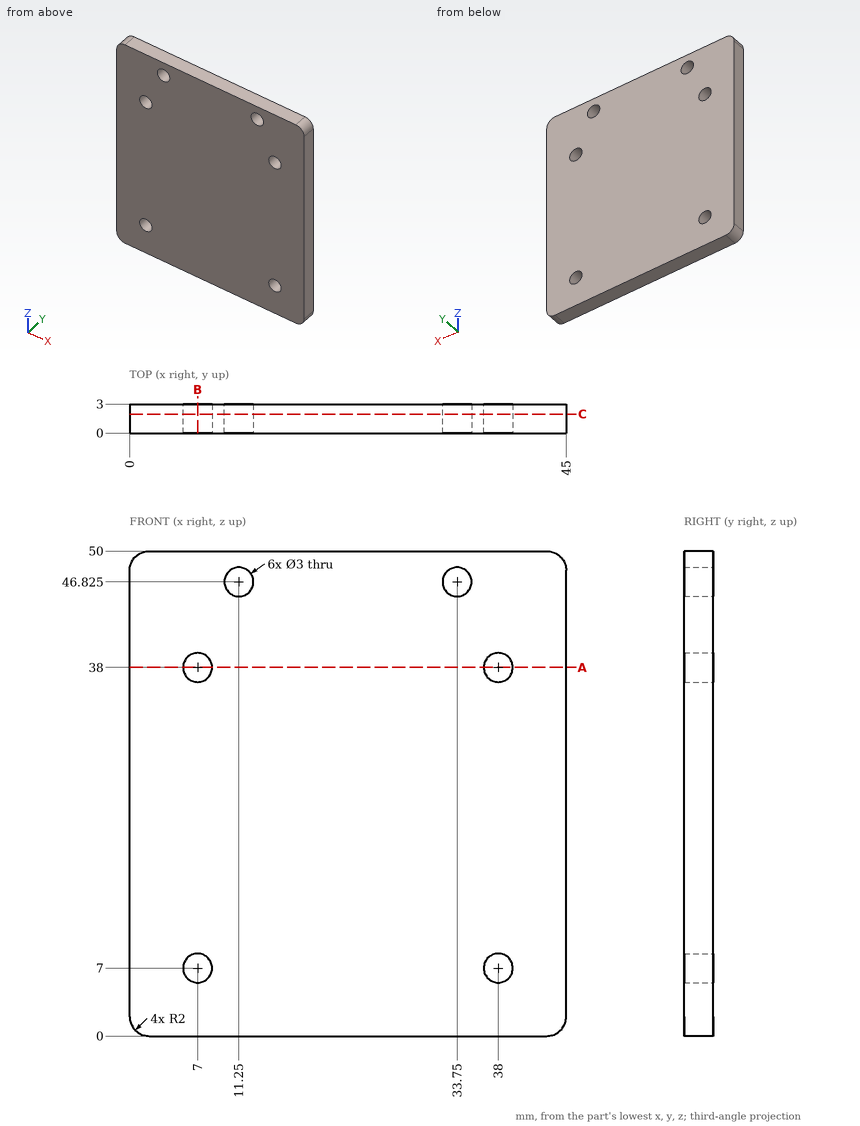
Can you work these out from the drawing? Everything is in mm from the part's minimum corner. Coordinates: 2 decimals unless noted, no trailing zeros. Loops run counter-clockwise (first coordinate to the right, second up) from the corner with the lowest first, then second, coordinate; pieces in that order, holes last. Notation, with made-up numbers: (-20, -33.5) - (11, -33.5) arc R14 cw to (11, -17.5) - close; hole circle Ø9 at (40.5, 53.5). An arc over 180 degrees is marked (long way). Answer as CSV lines item,"result".
Q1. For pin 1 (5 mm diameter, centred on x = 33.75, z = 46.825, fed in from +Y); pin 2 (2.5 mm diameter, centred on x = 38, z = 38, fed in from -Y), each with a flat end and sliding along its axis, tell me the tip position at first contact or that it passes through.
Response:
pin 1,"y = 3"
pin 2,"through"
Q2. If we section it at C-C, the plane y = 1.95: Write out the boundary of the cut face in (x, z) (3 decimals).
Response:
outline,"(0, 2) arc R2 ccw to (2, 0) - (43, 0) arc R2 ccw to (45, 2) - (45, 48) arc R2 ccw to (43, 50) - (2, 50) arc R2 ccw to (0, 48) - close; hole circle Ø3 at (7, 7); hole circle Ø3 at (7, 38); hole circle Ø3 at (11.25, 46.825); hole circle Ø3 at (33.75, 46.825); hole circle Ø3 at (38, 7); hole circle Ø3 at (38, 38)"
Q3. If we section it at A-A, the plane z = 38: Write out the boundary of the cut face in (x, y), and give its area (3 significant figures).
Response:
outline,"(0, 0) - (5.5, 0) - (5.5, 3) - (0, 3) - close; (8.5, 0) - (36.5, 0) - (36.5, 3) - (8.5, 3) - close; (39.5, 0) - (45, 0) - (45, 3) - (39.5, 3) - close"
area,"117 mm2"
Q4. If I drill on L1, parallel to Z at x = 38, y = 1.75; L2, parallel to Z at x = 37, y = 2.8; L3, parallel to Z at x = 33.75, y = 1.25 (3 decimals), over which ranges is the centre line in solid material (lowest first)? Write a range as [from, to].
Response:
L1,"[0, 5.5], [8.5, 36.5], [39.5, 50]"
L2,"[0, 5.88], [8.12, 36.88], [39.12, 50]"
L3,"[0, 45.325], [48.325, 50]"
Q5. If we section it at B-B, the plane x = 7: Write out the boundary of the cut face in (y, z).
Response:
outline,"(0, 0) - (3, 0) - (3, 5.5) - (0, 5.5) - close; (0, 8.5) - (3, 8.5) - (3, 36.5) - (0, 36.5) - close; (0, 39.5) - (3, 39.5) - (3, 50) - (0, 50) - close"
